The listing builds one solid part. Answer for the finished solid, in the listing's coordinates (mm). A direction names the side the tool comes from. Give positions to 0.01 mm unless a question says otherwise; leave off trailing zeros. Order: outer loops, then holes, each group sorted by start corner. A loop starts at its lowest first (then second) coordinate and runs counter-clockwise, first axis right, second up. Notation, with made-up numbers: M 37,57 L 90,57 A20 cw 90,76 Z; hole C 8,38.25 d11. An arc over 180 degrees is marked long. Answer as a JSON object with one key per item and string values. Group by question number.
```python
from build123d import *

# Parameters (mm, degrees)
SKETCH1_W           = 42
SKETCH1_H           = 42
BOSS_EXTRUDE1_DEPTH = 33.2
CHAMFER1_SIZE       = 4
SKETCH2_R           = 16
CUT_EXTRUDE1_DEPTH  = 0.5
SKETCH3_R           = 11
BOSS_EXTRUDE3_DEPTH = 2.5
SKETCH4_R           = 3.5
CUT_EXTRUDE2_DEPTH  = 2.5
SKETCH7_R           = 5.5
CUT_EXTRUDE4_DEPTH  = 4
SKETCH5_R           = 2.5
BOSS_EXTRUDE4_DEPTH = 21
CUT_EXTRUDE3_START  = -16
CUT_EXTRUDE3_DEPTH  = 16
CHAMFER2_SIZE       = 0.5
SKETCH8_R           = 1.6
CUT_EXTRUDE5_DEPTH  = 6
SKETCH9_W           = 8
SKETCH9_H           = 7
CUT_EXTRUDE6_DEPTH  = 4
FILLET1_R           = 1


with BuildPart() as part:
    # Sketch1 → Boss-Extrude1 (new body)
    with BuildSketch(Plane(origin=(0, 0, 0), x_dir=(1, 0, 0), z_dir=(0, 1, 0))):
        with Locations((21, 21)):
            Rectangle(SKETCH1_W, SKETCH1_H)
    extrude(amount=BOSS_EXTRUDE1_DEPTH)

    # Chamfer1
    chamfer1_edges = [part.edges().sort_by_distance(p)[0] for p in [
        (0, 16.6, -42),
        (42, 16.6, -42),
        (42, 16.6, 0),
        (0, 16.6, 0),
    ]]
    chamfer(chamfer1_edges, length=CHAMFER1_SIZE)

    # Sketch2 → Cut-Extrude1 (cut)
    with BuildSketch(Plane(origin=(0, 33.2, 0), x_dir=(1, 0, 0), z_dir=(0, 1, 0))):
        with Locations(Location((21, 21, 0), (0, 0, 270))):
            Circle(SKETCH2_R)
    extrude(amount=-CUT_EXTRUDE1_DEPTH, mode=Mode.SUBTRACT)

    # Sketch3 → Boss-Extrude3 (add)
    with BuildSketch(Plane(origin=(0, 32.7, 0), x_dir=(1, 0, 0), z_dir=(0, 1, 0))):
        with Locations(Location((21, 21, 0), (0, 0, 270))):
            Circle(SKETCH3_R)
    extrude(amount=BOSS_EXTRUDE3_DEPTH)

    # Sketch4 → Cut-Extrude2 (cut)
    with BuildSketch(Plane(origin=(0, 35.2, 0), x_dir=(1, 0, 0), z_dir=(0, 1, 0))):
        with Locations(Location((21, 21, 0), (0, 0, 270))):
            Circle(SKETCH4_R)
    extrude(amount=-CUT_EXTRUDE2_DEPTH, mode=Mode.SUBTRACT)

    # Sketch7 → Cut-Extrude4 (cut)
    with BuildSketch(Plane.XZ):
        with Locations(Location((21, -21.16858083, 0), (0, 0, 270))):
            Circle(SKETCH7_R)
    extrude(amount=-CUT_EXTRUDE4_DEPTH, mode=Mode.SUBTRACT)

    # Sketch5 → Boss-Extrude4 (add)
    with BuildSketch(Plane(origin=(0, 32.7, 0), x_dir=(1, 0, 0), z_dir=(0, 1, 0))):
        with Locations(Location((21, 21, 0), (0, 0, 90))):
            Circle(SKETCH5_R)
    extrude(amount=BOSS_EXTRUDE4_DEPTH)

    # Sketch6 → Cut-Extrude3 (cut)
    with BuildSketch(Plane(origin=(0, 53.7, 0), x_dir=(1, 0, 0), z_dir=(0, 1, 0)).offset(CUT_EXTRUDE3_START)):
        with BuildLine():
            Line((19.5, 23), (22.5, 23))
            ThreePointArc((22.5, 23), (21, 23.5), (19.5, 23))
        make_face()
    extrude(amount=CUT_EXTRUDE3_DEPTH, mode=Mode.SUBTRACT)

    # Chamfer2
    chamfer2_edges = [part.edges().sort_by_distance(p)[0] for p in [
        (21, 53.7, -18.5),
        (21, 53.7, -23),
    ]]
    chamfer(chamfer2_edges, length=CHAMFER2_SIZE - 0.0001)  # a hair under: the kernel refuses the full size

    # Sketch8 → Cut-Extrude5 (cut)
    with BuildSketch(Plane(origin=(0, 33.2, 0), x_dir=(1, 0, 0), z_dir=(0, 1, 0))):
        with Locations(Location((5.5, 36.5, 0), (0, 0, 270))):
            Circle(SKETCH8_R)
        with Locations(Location((36.5, 36.5, 0), (0, 0, 270))):
            Circle(SKETCH8_R)
        with Locations(Location((36.5, 5.5, 0), (0, 0, 270))):
            Circle(SKETCH8_R)
        with Locations(Location((5.5, 5.5, 0), (0, 0, 270))):
            Circle(SKETCH8_R)
    extrude(amount=-CUT_EXTRUDE5_DEPTH, mode=Mode.SUBTRACT)

    # Sketch9 → Cut-Extrude6 (cut)
    with BuildSketch(Plane(origin=(0, 0, -42), x_dir=(-1, 0, 0), z_dir=(0, 0, -1))):
        with Locations((-21, 5.8)):
            Rectangle(SKETCH9_W, SKETCH9_H)
    extrude(amount=-CUT_EXTRUDE6_DEPTH, mode=Mode.SUBTRACT)

    # Fillet1
    fillet1_edges = [part.edges().sort_by_distance(p)[0] for p in [
        (0, 0, -21),
        (0, 16.6, -4),
        (0, 16.6, -38),
        (21, 0, -42),
        (42, 0, -21),
        (21, 0, 0),
        (40, 0, -2),
        (2, 0, -2),
        (40, 0, -40),
        (2, 0, -40),
        (38, 16.6, -42),
        (4, 16.6, -42),
        (42, 16.6, -4),
        (42, 16.6, -38),
        (38, 16.6, 0),
        (4, 16.6, 0),
        (21, 0, -15.66858083),
    ]]
    fillet(fillet1_edges, radius=FILLET1_R)


solid = part.part
```
Item 1: Section A-A (y = 16) is taken. Determine the outline of the cut face in (x, z).
Item 2: Section C-C (x = 34) is taken. Determine the outline of the cut face in (y, z).
Item 3: Determine the mould class of faces 1 (the cylindrical face through (39.822, 0.301, -2.226)), 2 (the flat face through (21, 2.3, -40)), 3 (the flat face through (6, 27.2, -6)), 4 (the flat face through (17, 6, -40)) for opening direction Y: released by +Y, released by -Y, zero draft, split by the parting line, or undercut.
Item 4: Consider probe 1 along X at (y, z) = (31.4, -5.5); probe 2 along X at (y, z) = (33, -21); probe 3 along X at (y, z) = (34.1, -21). Determine where each line is inside the solid, lowest interval first. Write a range as from..to.
Item 5: A tool of negligible diameter and unlimited length cuts with its end or side. For faces 5 (the flat face through (21, 9.3, -40)), 6 (the flat face through (40, 17, -2)), 7 (the flat face through (6, 27.2, -37)), 8 (the cylindrical face through (24.7, 2.5, -17.1)), 9 (the flat face through (21, 45, -23)), from which of +Z, -Z, +X, -X, +Y, -Y can it reach the whole face along a straight path? Write none if from no direction.
Item 6: Section B-B (z = -6) is taken. Determine the outline of the cut face in (x, y).
Item 7: Flat-ended cylindrical pins translate along their axes: P1, Ø2.5, axis at x = 20.5, y = 44, coming from the -Z side; P2, Ø2, axis at x = 19.5, y = 7.5, coming from the -Z side; P3, Ø1.6, axis at x = 6, z = -6, coming from the +Y side; P4, Ø5, axis at x = 36.5, z = -36.5, coming from the -Y side. Find the tip coordinate at first contact, or state that the pin passes through.
Item 8: Section D-D (y = 5.5) is taken. Determine the outline of the cut face in (x, z).
Values found:
{
 "1": {"outline": "M 0,-37.59 A1 ccw 0.29,-38.29 L 3.71,-41.71 A1 ccw 4.41,-42 L 37.59,-42 A1 ccw 38.29,-41.71 L 41.71,-38.29 A1 ccw 42,-37.59 L 42,-4.41 A1 ccw 41.71,-3.71 L 38.29,-0.29 A1 ccw 37.59,0 L 4.41,0 A1 ccw 3.71,-0.29 L 0.29,-3.71 A1 ccw 0,-4.41 Z"},
 "2": {"outline": "M 0,-41 A1 ccw 1,-42 L 33.2,-42 L 33.2,-30.33 L 32.7,-30.33 L 32.7,-11.67 L 33.2,-11.67 L 33.2,0 L 1,0 A1 ccw 0,-1 Z"},
 "3": {"face 1": "released by -Y", "face 2": "undercut", "face 3": "released by +Y", "face 4": "undercut"},
 "4": {"probe 1": "x = 0..3.9, 7.1..34.9, 38.1..42", "probe 2": "x = 0..5, 10..17.5, 18.5..23.5, 24.5..32, 37..42", "probe 3": "x = 10..17.5, 18.5..23.5, 24.5..32"},
 "5": {"face 5": "-Z", "face 6": "+Z, +X, +Y, -Y", "face 7": "+Y", "face 8": "-Y", "face 9": "-Z, +X, -X, +Y"},
 "6": {"outline": "M 0,1 A1 ccw 1,0 L 41,0 A1 ccw 42,1 L 42,33.2 L 38.02,33.2 L 38.02,27.2 L 34.98,27.2 L 34.98,33.2 L 26.57,33.2 L 26.57,32.7 L 15.43,32.7 L 15.43,33.2 L 7.02,33.2 L 7.02,27.2 L 3.98,27.2 L 3.98,33.2 L 0,33.2 Z"},
 "7": {"P1": "stops at z = -23", "P2": "stops at z = -38", "P3": "stops at y = 27.2", "P4": "stops at y = 0"},
 "8": {"outline": "M 0,-37.59 A1 ccw 0.29,-38.29 L 3.71,-41.71 A1 ccw 4.41,-42 L 17,-42 L 17,-38 L 25,-38 L 25,-42 L 37.59,-42 A1 ccw 38.29,-41.71 L 41.71,-38.29 A1 ccw 42,-37.59 L 42,-4.41 A1 ccw 41.71,-3.71 L 38.29,-0.29 A1 ccw 37.59,0 L 4.41,0 A1 ccw 3.71,-0.29 L 0.29,-3.71 A1 ccw 0,-4.41 Z"}
}
